```python
from build123d import *

# Parameters (mm, degrees)
SKETCH_1_W          = 14
SKETCH_1_H          = 16
EXTRUDE_1_DEPTH     = 1.8
SHELL_1_T           = -0.2
CUT_EXTRUDE_2_DEPTH = 0.3


with BuildPart() as part:
    # 草图1 → 拉伸1 (new body)
    with BuildSketch(Plane(origin=(0, 0, 0), x_dir=(1, 0, 0), z_dir=(0, 1, 0))):
        Rectangle(SKETCH_1_W, SKETCH_1_H)
    extrude(amount=EXTRUDE_1_DEPTH)

    # 抽壳1
    shell_1_openings = [part.faces().sort_by_distance(p)[0] for p in [
        (0, 0.9, 8),
    ]]
    offset(amount=SHELL_1_T, openings=shell_1_openings, kind=Kind.INTERSECTION)

    # 草图2 → 切除-拉伸2 (cut)
    with BuildSketch(Plane.XZ):
        with BuildLine():
            Line((7, 8), (-7, 8))
            ThreePointArc((-7, 8), (0, 7.20758668), (7, 8))
        make_face()
    extrude(amount=-CUT_EXTRUDE_2_DEPTH, mode=Mode.SUBTRACT)


solid = part.part
```
Part model, mm, in its own coordinate system. A direction names the side the tool comes from. Round coordinates to 2 decimals unless told otherwise and drop trailing zeros. Loops run counter-clockwise (first coordinate to the right, second up) from the corner with the lowest first, then second, coordinate; pieces in that order, holes last.
Item 1: Cut at A-A, the plane z = 3. Give the cut face in (x, y).
Item 2: 3-axis set-ups, long thin cutter, end or side, ignore diameter. For faces 5 (the face through (0, 1, -8)), 6 (the face through (-6.8, 1, 0)): which of +Z, -Z, +X, -X, +Y, -Y reach the whole face in a straight line?
Item 3: Cut at B-B, the plane y = 1.4. Give the cut face in (x, z), then the cut area to 3 significant figures.
Item 4: Mould opens along X. For faces 1 (the face through (0, 0, 0)), 2 (the face through (0, 1.6, 0)), 3 (the face through (7, 1, 0)), 4 (the face through (-7, 1, 0)) say: +X half, -X half, draft (parallel to the pull), parting line (faces both ways), or undercut.
Item 5: Cut at C-C, the plane x = 2.75. Give the cut face in (y, z), then the cut area to 3 significant figures.
Item 6: Drill centre lines: line 1 (Y direction, x = 1.75, z = -1.75); line 2 (X direction, y = 1.05, z = 4.25); line 3 (Z direction, x = 0.25, y = 1.1). Where is each one in solid material? Low to high.
A:
1. outline: (-7, 0) - (7, 0) - (7, 1.8) - (-7, 1.8) - close; hole (-6.8, 0.2) - (6.8, 0.2) - (6.8, 1.6) - (-6.8, 1.6) - close
2. face 5: -Z, +X, -X, +Y, -Y
2. face 6: +Z
3. outline: (-7, -8) - (7, -8) - (7, 8) - (6.8, 8) - (6.8, -7.8) - (-6.8, -7.8) - (-6.8, 8) - (-7, 8) - close
3. area: 9.12 mm2
4. face 1: draft
4. face 2: undercut
4. face 3: +X half
4. face 4: -X half
5. outline: (0, -8) - (1.8, -8) - (1.8, 8) - (1.6, 8) - (1.6, -7.8) - (0.2, -7.8) - (0.2, 7.33) - (0, 7.33) - close
5. area: 6.55 mm2
6. line 1: y = 0 to 0.2, 1.6 to 1.8
6. line 2: x = -7 to -6.8, 6.8 to 7
6. line 3: z = -8 to -7.8
